Check sheet for the modelled part. Datum: model origin and axes. Units: mm. Round coordinates to 2 decimals unless told otherwise and drop trailing zeros. Write each loop counter-clockwise with the first axis right and the second up, starting at its lowest first coordinate (ties: lowest second). Pieces come first, ordered by that corner, then holes.
Item 1: Cross-section at A-A on z = 2.4. Enter the section's corners in (x, y).
Item 2: Material ranges on line 1 (Y direction, x = 40.5, z = 1.85); line 2 (X direction, y = 20, z = 3.9); line 3 (X direction, y = 16.5, z = 1.4), recorded low to high.
Item 3: Cross-section at C-C on y = 80. Enter the section's corners in (x, z).
Item 4: Cross-section at D-D on x = 8. Enter the section's corners in (y, z).
Item 5: Cross-section at B-B on x = 40.5. Enter the section's corners in (y, z), plus the area to 3 significant figures.
Item 6: Go/stop test with flat-tipped pins: pin 1 Ø14.5 at (x, y) = (40.5, 80) entering from +Z; pin 2 Ø1 at (y, z) = (-60, 1.5) entering from +X; pin 3 Ø3 at (x, z) = (23, 3.5) entering from +Y. Record where each tip stops, or that it passes through.
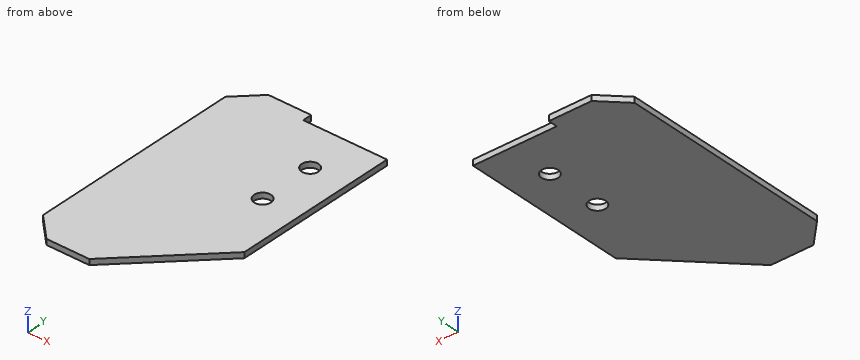
Autodesk Fusion 360 part; units mm, degrees
sketch "スケッチ1" plane through (0, 0, 0) normal (0, 0, 1) x (1, 0, 0)
  line L0 (-9.5, 140) -> (-80.5, 140)
  line L1 (-80.5, 140) -> (-80.5, -140)
  line L2 (-80.5, -140) -> (-9.5, -140)
  line L3 (80.5, -50) -> (80.5, 130)
  line L4 (74.75, 130) -> (-80.5, -140) construction
  line L5 (-80.5, 140) -> (47.6429, -82.8571) construction
  line L6 (-9.5, 140) -> (-9.5, 130)
  line L7 (-9.5, 130) -> (80.5, 130)
  line L8 (-80.5, -140) -> (-9.5, -140) construction
  line L9 (80.5, -50) -> (-9.5, -140)
  dimension "d2" = 280
  dimension "d5" = 71
extrude "押し出し1" add sketch "スケッチ1" along normal blind 6
chamfer "面取り1" distance 25 angle 45 2 edges at (-80.5, -140, 3) (-80.5, 140, 3)
sketch "スケッチ2" plane through (0, 0, 6) normal (0, 0, 1) x (-1, 0, 0)
  line L0 (55.5, -140) -> (80.5, -115)
  line L1 (80.5, -115) -> (80.5, 115)
  line L2 (80.5, 115) -> (55.5, 140)
  line L3 (55.5, 140) -> (9.5, 140)
  line L4 (9.5, 140) -> (-80.5, 50)
  line L5 (-80.5, 50) -> (-80.5, -130)
  line L6 (-80.5, -130) -> (9.5, -130)
  line L7 (9.5, -130) -> (9.5, -140)
  line L8 (9.5, -140) -> (55.5, -140)
  line L9 (-80.5, -130) -> (-40.5, -130) construction
  line L10 (-40.5, -130) -> (-40.5, -80) construction
  line L11 (-40.5, -80) -> (-80.5, -80) construction
  line L12 (-80.5, -80) -> (-80.5, -130) construction
  line L13 (-40.5, -80) -> (-40.5, -20) construction
  point P0 (-40.5, -80)
  point P1 (-40.5, -20)
  dimension "d10" = 40
  dimension "d11" = 50
  dimension "d12" = 60
hole "穴1" at (40.5, 80, 6) at (40.5, 20, 6) direction (0, 0, -1) diameter 18 end through all
equation "d5 = 25 mm + 46 mm"
Response values:
1. outline: (-80.5, -115) - (-55.5, -140) - (-9.5, -140) - (80.5, -50) - (80.5, 130) - (-9.5, 130) - (-9.5, 140) - (-55.5, 140) - (-80.5, 115) - close; hole circle Ø18 at (40.5, 20); hole circle Ø18 at (40.5, 80)
2. line 1: y = -90 to 11, 29 to 71, 89 to 130
2. line 2: x = -80.5 to 31.5, 49.5 to 80.5
2. line 3: x = -80.5 to 32.21, 48.79 to 80.5
3. outline: (-80.5, 0) - (31.5, 0) - (31.5, 6) - (-80.5, 6) - close; (49.5, 0) - (80.5, 0) - (80.5, 6) - (49.5, 6) - close
4. outline: (-122.5, 0) - (130, 0) - (130, 6) - (-122.5, 6) - close
5. outline: (-90, 0) - (11, 0) - (11, 6) - (-90, 6) - close; (29, 0) - (71, 0) - (71, 6) - (29, 6) - close; (89, 0) - (130, 0) - (130, 6) - (89, 6) - close
5. area: 1,100 mm2
6. pin 1: passes through
6. pin 2: stops at x = 71
6. pin 3: stops at y = 130
